Autodesk Inventor part; units mm, degrees
ref_plane "YZ Plane" through (0, 0, 0) normal (1, 0, 0) x (0, 1, 0)
ref_plane "XZ Plane" through (0, 0, 0) normal (0, 1, 0) x (-1, 0, 0)
ref_plane "XY Plane" through (0, 0, 0) normal (0, 0, 1) x (1, 0, 0)
sketch "Sketch2" plane through (0, 0, 0) normal (0, 1, 0) x (-1, 0, 0)
  line L0 (0, 0) -> (-25.4, 0)
  line L1 (-25.4, 0) -> (0, 0)
  line L2 (0, 0) -> (0, -50.8)
  line L3 (0, -50.8) -> (-25.4, -50.8)
  line L4 (-25.4, -50.8) -> (-25.4, 0)
  line L5 (-22.225, -47.625) -> (-3.175, -47.625)
  line L6 (-3.175, -47.625) -> (-3.175, -3.175)
  line L7 (-3.175, -3.175) -> (-22.225, -3.175)
  line L8 (-22.225, -3.175) -> (-22.225, -47.625)
  dimension "d2" = 25.4
  dimension "d3" = 50.8
  dimension "d4" = 19.05
  dimension "d5" = 44.45
  dimension "d6" = 3.175
  dimension "d7" = 3.175
extrude "Extrusion1" add sketch "Sketch2" along normal blind 1219.2
sketch "Sketch3" plane through (25.4, 0, -50.8) normal (0, 0, -1) x (-1, 0, 0)
  line L0 (25.4, 1219.2) -> (25.4, 609.6) construction
  line L1 (25.4, 0) -> (25.4, 1219.2)
  line L2 (25.4, 609.6) -> (0, 609.6) construction
  line L3 (0, 0) -> (0, 1219.2)
  line L4 (12.7, 609.6) -> (12.7, 622.3) construction
  circle A0 centre (12.7, 622.3) radius 3.175
  line L5 (12.7, 609.6) -> (12.7, 596.9) construction
  circle A1 centre (12.7, 596.9) radius 3.175
  dimension "d10" = 1219.2
  dimension "d11" = 609.6
  dimension "d12" = 12.7
  dimension "d13" = 6.35
extrude "Extrusion2" cut sketch "Sketch3" against normal blind 1219.2
sketch "Sketch4" plane through (0, 0, -50.8) normal (-1, 0, 0) x (0, 0, 1)
  line L0 (3.175, 1219.2) -> (47.625, 1219.2)
  line L1 (25.4, 1219.2) -> (25.4, 1190.625)
  circle A0 centre (25.4, 1190.625) radius 14.2875
  point P0 (50.8, 0)
  dimension "d16" = 28.575
  dimension "d17" = 28.575
extrude "Extrusion3" cut sketch "Sketch4" against normal blind 6.35
sketch "Sketch5" plane through (25.4, 0, 0) normal (1, 0, 0) x (0, 0, -1)
  line L0 (47.625, 0) -> (3.175, 0) construction
  line L1 (25.4, 0) -> (25.4, 114.3) construction
  line L2 (50.8, 0) -> (50.8, 1219.2) construction
  line L3 (50.8, 0) -> (38.1, 0) construction
  circle A0 centre (38.1, 114.3) radius 1.5875
  circle A1 centre (12.7, 114.3) radius 1.5875
  line L4 (0, 0) -> (0, 1219.2) construction
  line L5 (0, 127) -> (50.8, 127) construction
  circle A2 centre (38.1, 139.7) radius 1.5875
  circle A3 centre (12.7, 139.7) radius 1.5875
  dimension "d20" = 114.3
  dimension "d21" = 12.7
  dimension "d22" = 3.175
hole "Hole1" at (25.4, 139.7, -12.7) at (25.4, 114.3, -12.7) at (25.4, 114.3, -38.1) at (25.4, 139.7, -38.1) direction (-1, 0, 0) diameter 3.175 depth 3.175 tip angle 118
sketch "Sketch7" plane through (0, 0, -50.8) normal (-1, 0, 0) x (0, 0, 1)
  circle A0 centre (25.4, 19.05) radius 14.7752
  point P0 (50.8, 0)
  point P1 (39.6875, 22.815)
hole "Hole3" at (0, 19.05, -25.4) direction (1, 0, 0) diameter 28.575 depth 3.175 tip angle 118
sketch "Sketch8" plane through (25.4, 0, 0) normal (1, 0, 0) x (0, 0, -1)
  point P0 (0, 0)
sketch "Sketch9" plane through (0, 0, 0) normal (0, 0, 1) x (1, 0, 0)
  circle A0 centre (12.7, 596.9) radius 3.175
  line L0 (12.7, 596.9) -> (12.7, 0)
  point P0 (0, 0)
  dimension "d48" = 596.9
sketch "Sketch10" plane through (0, 0, -50.8) normal (-1, 0, 0) x (0, 0, 1)
  circle A0 centre (25.4, 596.9) radius 3.175
  line L0 (50.8, 0) -> (50.8, 1219.2)
  line L1 (50.8, 0) -> (0, 0)
  line L2 (0, 0) -> (0, 1219.2)
  line L3 (0, 609.6) -> (50.8, 609.6)
  line L4 (50.8, 0) -> (50.8, 1219.2)
  line L5 (0, 1219.2) -> (50.8, 1219.2)
  circle A1 centre (25.4, 622.3) radius 3.175
  dimension "d49" = 6.35
  dimension "d50" = 25.4
  dimension "d51" = 596.9
  dimension "d52" = 609.6
hole "Hole4" at (0, 622.3, -25.4) at (0, 596.9, -25.4) direction (1, 0, 0) diameter 6.35 depth 25.4 tip angle 118
properties part number "main beam" material "Aluminum 6061"
Part model, mm, in its own coordinate system. A direction names the side the tool comes from. Give positions to 0.01 mm unless a question says otherwise; leave off trailing zeros. Write each loop counter-clockwise with the first axis right and the second up, starting at its lowest first coordinate (ties: lowest second). Pieces come first, ordered by that corner, then holes. Notation, with made-up numbers: M 24,49.25 L 33,49.25 A12 cw 33,62.25 Z; hole C 49,27 d3. An arc over 180 degrees is marked long. Use CSV: the item, a comma, the result in double quotes.
Item 1: Drill centre lines: probe 1 along Y at (x, z) = (23.3, -38.1); probe 2 along Y at (x, z) = (1.8, -25.4) (1 decimal); probe 3 along Z at (x, y) = (6.5, 1068.5) (3 decimals). Where is each one in solid material? Low to high.
Taken from the geometry:
probe 1,"y = 0 to 112.71, 115.89 to 138.11, 141.29 to 1219.2"
probe 2,"y = 0 to 4.8, 33.3 to 593.7, 600.1 to 619.1, 625.5 to 1176.3, 1204.9 to 1219.2"
probe 3,"z = -50.8 to -47.625, -3.175 to 0"
Item 2: Pin check, flat tip, straight feed: P1, Ø15, axis at x = 11.5, y = 390.5, coming from the +Z side. Stop position of the tip, or through.
Taken from the geometry:
P1,"stops at z = 0"
Item 3: Slice it at A-A on y = 573. Write the cut outline in (x, z) (3 decimals).
Taken from the geometry:
outline,"M 0,-50.8 L 25.4,-50.8 L 25.4,0 L 0,0 Z; hole M 3.175,-47.625 L 22.225,-47.625 L 22.225,-3.175 L 3.175,-3.175 Z"
Item 4: Which spindle directions (+Z, -Z, +X, -X, +Y, -Y) get a long thin tool onto all of the face, cutting with end or side? Do faces 1 (the face through (23, 1219.2, -27)), 2 (the face through (22.225, 601, -25)), 3 (the face through (1.57, 1200.28, -35.93)). Say none if no direction does.
Taken from the geometry:
face 1,"+Z, -Z, +X, -X, +Y"
face 2,"+Y, -Y"
face 3,"-X"
Item 5: Pull direction Z, two halves, no side cores. Call faces 4 (the face through (0, 601, -25)), 5 (the face through (1.61, 9.394, -35.93)), 6 (the face through (13, 601, 0)): +Z half, -Z half, draft (parallel to the pull), parting line (faces both ways), or undercut.
Taken from the geometry:
face 4,"draft"
face 5,"undercut"
face 6,"+Z half"
